from build123d import *

# Parameters (mm, degrees)
SKETCH1_R           = 0.8382
BOSS_EXTRUDE1_DEPTH = 19.05
CUT_EXTRUDE1_START  = 76.2
SKETCH2_R           = 1.8034
SKETCH2_W           = 2.9464
SKETCH2_H           = 6.35
CUT_EXTRUDE1_DEPTH  = 127


with BuildPart() as part:
    # Sketch1 → Boss-Extrude1 (new body)
    with BuildSketch(Plane.XY):
        with BuildLine():
            Line((-11.0348776, 1.636724806), (-11.0348776, 2.271724806))
            Line((-11.0348776, 2.271724806), (-4.296180386, 2.271724806))
            ThreePointArc((-4.296180386, 2.271724806), (-2.400761669, 4.41475324), (-3.0846776, 1.636724806))
            Line((-3.0846776, 1.636724806), (-11.0348776, 1.636724806))
        make_face()
        with Locations((-3.0846776, 3.109924806)):
            Circle(SKETCH1_R, mode=Mode.SUBTRACT)
    extrude(amount=BOSS_EXTRUDE1_DEPTH)

    # Sketch2 → Cut-Extrude1 (cut)
    with BuildSketch(Plane(origin=(0, 2.271724806, 0), x_dir=(1, 0, 0), z_dir=(0, 1, 0)).offset(CUT_EXTRUDE1_START)):
        with Locations((-7.665528993, -3.9624)):
            Circle(SKETCH2_R)
        with Locations((-7.665528993, -15.0876)):
            Circle(SKETCH2_R)
        with Locations((-3.0846776, -3.175)):
            Rectangle(SKETCH2_W, SKETCH2_H)
        with Locations((-3.0846776, -15.875)):
            Rectangle(SKETCH2_W, SKETCH2_H)
    extrude(amount=-CUT_EXTRUDE1_DEPTH, mode=Mode.SUBTRACT)


solid = part.part
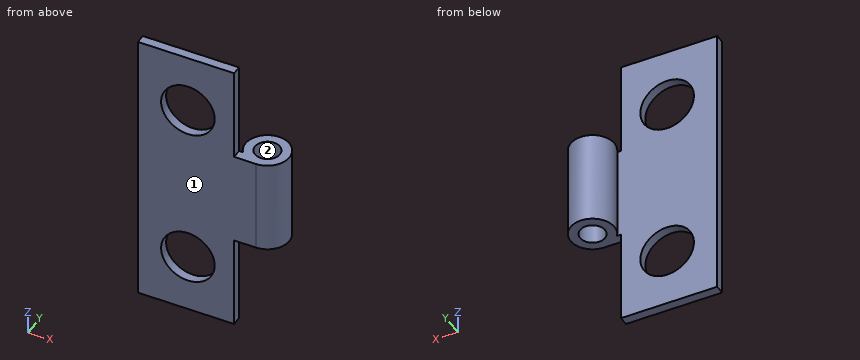
Could you check a few things on this model? Use its own coordinates, in mm. Face numbers are marked on the shaded views. Give positions to 0.01 mm unless a question says otherwise; leave off trailing zeros. Write each loop counter-clockwise with the first axis right and the second up, starting at its lowest first coordinate (ties: lowest second). Pieces come first, ordered by that corner, then holes. Notation, with made-up numbers: (89.5, -39.75) - (133.5, -39.75) arc R21 ccw to (133.5, -24.75) - close; hole circle Ø5 at (-39, 31). An arc over 180 degrees is marked (long way). Use CSV: the item, a comma, the result in double quotes. Start each with the question number.
Item 1: I want a section at C-C, the plane y = 2.65. Please give me the cut outline in (x, z), then the cut area to 4 significant figures.
Item 2: If I drill on line 1 along Y through (x, z) = (-3, 9.5); line 2 along X through (y, z) = (1.95, 4); line 3 along X through (y, z) = (2.2, 1), over which ranges is the centre line in solid material (lowest first)?
Item 3: I'm going to push a flat-ended pin straight in: pin 1 (1.5 mm diameter, centred on x = -8, y = 4, fed in from +Z). Where does the tip first touch, or does it pass through?
Item 4: If we mould it in two halves opening along X, with no side actions, what happens to the marked faces 1 and 2? For each: pulls with the +X half, pulls with the -X half, needs draft (parallel to the pull), parting line crosses it, or undercut.
Item 5: I want a section at A-A, the plane x = -7.5. Please give me the cut outline in (y, z).
Item 6: I want a section at D-D, the plane y = 1.85. Please give me the cut outline in (x, z).
Item 7: I want a section at B-B, the plane z = 4.5. Please give me the cut outline in (x, y), then the cut area to 3 significant figures.
Findings:
1,outline,"(-4.48, 6.35) - (-3.79, 6.35) - (-3.79, 12.7) - (-4.48, 12.7) - close; (-2.38, 6.35) - (-1.69, 6.35) - (-1.69, 12.7) - (-2.38, 12.7) - close"
1,area,"8.875 mm2"
2,line 1,"y = 1.64 to 2.28, 3.94 to 4.58"
2,line 2,"x = -11.03 to -9.47, -5.86 to -4.56"
2,line 3,"x = -11.03 to -4.56"
3,pin 1,"passes through"
4,face 1,"needs draft"
4,face 2,"undercut"
5,outline,"(1.64, 0) - (2.27, 0) - (2.27, 2.17) - (1.64, 2.17) - close; (1.64, 5.76) - (2.27, 5.76) - (2.27, 13.29) - (1.64, 13.29) - close; (1.64, 16.88) - (2.27, 16.88) - (2.27, 19.05) - (1.64, 19.05) - close"
6,outline,"(-11.03, 0) - (-4.56, 0) - (-4.56, 6.35) - (-2.32, 6.35) - (-2.32, 12.7) - (-4.56, 12.7) - (-4.56, 19.05) - (-11.03, 19.05) - close; hole circle Ø3.61 at (-7.67, 3.96); hole circle Ø3.61 at (-7.67, 15.09)"
7,outline,"(-11.03, 1.64) - (-9.39, 1.64) - (-9.39, 2.27) - (-11.03, 2.27) - close; (-5.94, 1.64) - (-4.56, 1.64) - (-4.56, 2.27) - (-5.94, 2.27) - close"
7,area,"1.93 mm2"
